Answer from the drawing. Dimensions are ordinates in mm from the lowest x, y and z of the part. Round coordinates to 2 decimals unless told otherwise and drop trailing zeros. Write each loop counter-clockwise with the first axis right and the second up, starting at its lowest first coordinate (ties: lowest second). Pieces come first, ordered by that corner, then holes. Notation, with made-up numbers: (86.5, 65.5) - (133.5, 65.5) arc R10 cw to (133.5, 77.5) - close; hole circle Ø6 at (-23, 0.5). An arc over 180 degrees is marked (long way). Answer as CSV lines item,"result". Start each with the question number.
1) Consider line 1 along Z through (x, y) = (104, 92); line 2 along Y through (x, z) = (24.5, 52.5); line 3 along Y through (x, z) = (130, 48.5). Determine where each line is inside the solid, lowest interval first.
2) Find section C-C on z = 40.5. Determine the outline of the cut face in (x, y), then the cut area to 3 significant figures.
3) Each of these flat-tipped pins is pushed along its axis until it touches: pin 1 (10 mm diameter, centred on x = 83.5, z = 59, fed in from +Y); pin 2 (2 mm diameter, centred on x = 66, z = 60, fed in from +Y); pin 3 (3 mm diameter, centred on x = 78, y = 76, fed in from +Z). Where does it stop, or does it pass through?
4) Find section B-B on y = 70. Determine the outline of the cut face in (x, z), then the cut area to 3 significant figures.
5) Find section A-A on x = 52.5. Determine the outline of the cut face in (y, z).
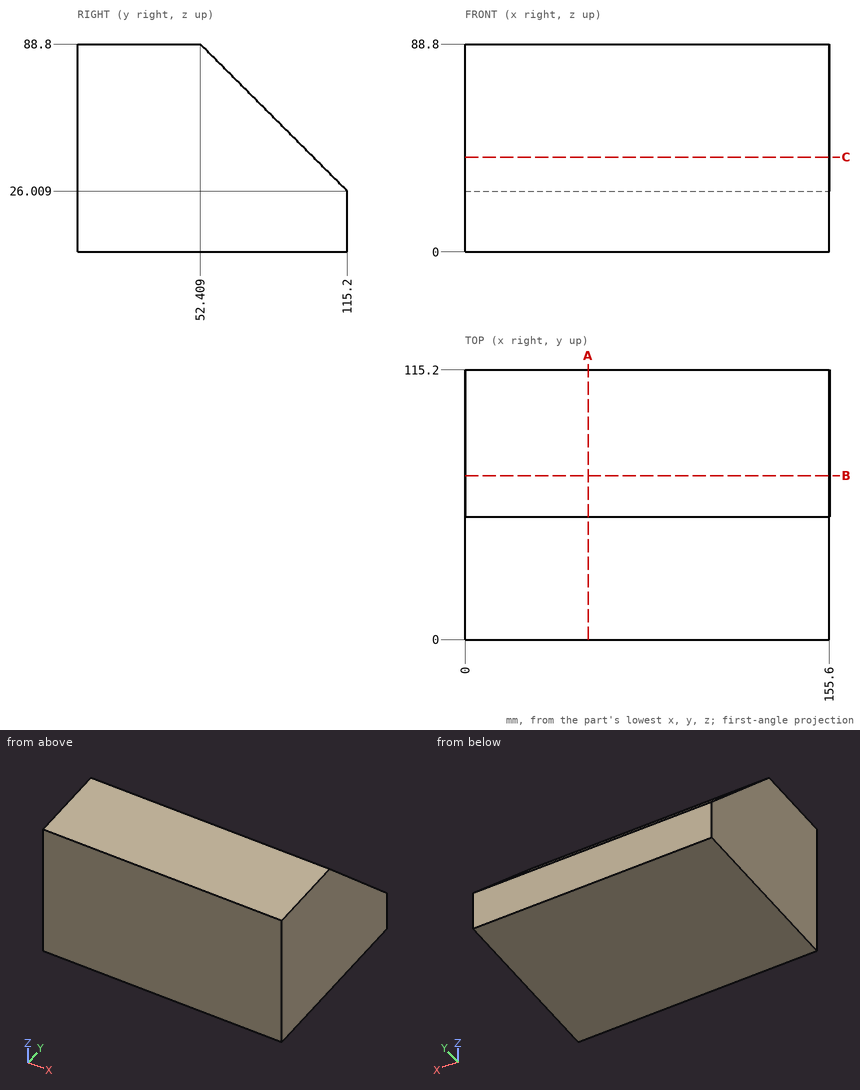
Check values:
1,line 1,"z = 0 to 49.21"
1,line 2,"y = 0 to 88.71"
1,line 3,"y = 0 to 92.71"
2,outline,"(0, 0) - (155.6, 0) - (155.6, 100.71) - (0, 100.71) - close"
2,area,"15,700 mm^2"
3,pin 1,"stops at y = 87.21"
3,pin 2,"stops at y = 82.21"
3,pin 3,"stops at z = 66.71"
4,outline,"(0, 0) - (155.6, 0) - (155.6, 71.21) - (0, 71.21) - close"
4,area,"11,100 mm^2"
5,outline,"(0, 0) - (115.2, 0) - (115.2, 26.01) - (52.41, 88.8) - (0, 88.8) - close"
